Autodesk Inventor part; units mm, degrees
ref_plane "YZ Plane" through (0, 0, 0) normal (1, 0, 0) x (0, 1, 0)
ref_plane "XZ Plane" through (0, 0, 0) normal (0, 1, 0) x (-1, 0, 0)
ref_plane "XY Plane" through (0, 0, 0) normal (0, 0, 1) x (1, 0, 0)
sketch "Esboço1" plane through (0, 0, 0) normal (0, 0, 1) x (1, 0, 0)
  line L0 (0, 0) -> (22, 0)
  line L1 (22, 0) -> (22, 20)
  line L2 (22, 20) -> (0, 20)
  line L3 (0, 20) -> (0, 0)
  dimension "d0" = 22
  dimension "d1" = 20
extrude "Extrusão1" add sketch "Esboço1" along normal blind 50
sketch "Esboço2" plane through (0, 0, 0) normal (0, -1, 0) x (1, 0, 0)
  line L0 (0, 0) -> (0, 50)
  line L1 (22, 50) -> (0, 50)
  point P0 (11, 15.5027)
  dimension "d20" = 11
  dimension "d35" = 34.4973
hole "Furo1" at (11, 0, 15.5027) direction (0, 1, 0) diameter 15 end through all
fillet "Arredondamento1" radius 5 4 edges at (22, 10, 0) (0, 10, 0) (0, 10, 50) (22, 10, 50)
sketch "Esboço4" plane through (5, 20, 0) normal (0, 1, 0) x (1, 0, 0)
  line L0 (12, -50) -> (0, -50)
  line L1 (6, -50) -> (6, -25)
  line L2 (1, -50) -> (11, -50)
  line L3 (11, -50) -> (11, -25)
  line L4 (11, -25) -> (1, -25)
  line L5 (1, -25) -> (1, -50)
  line L6 (1, -50) -> (11, -25) construction
  line L7 (11, -50) -> (1, -25) construction
  point P0 (-5, 0)
  point P1 (6, -37.5)
  dimension "d22" = 25
  dimension "d23" = 10
extrude "Extrusão2" cut sketch "Esboço4" against normal through all
sketch "Esboço5" plane through (16, 20, 25) normal (-1, 0, 0) x (0, 0, 1)
  line L0 (25, -20) -> (25, 0)
  point P0 (-25, -20)
  point P1 (20, -10)
  point P2 (10, -10)
  dimension "d33" = 5
  dimension "d34" = 10
hole "Furo3" at (16, 10, 45) at (16, 10, 35) direction (1, 0, 0) diameter 3 end through all both
properties part number "Base 1 LMU8_3DPrint"
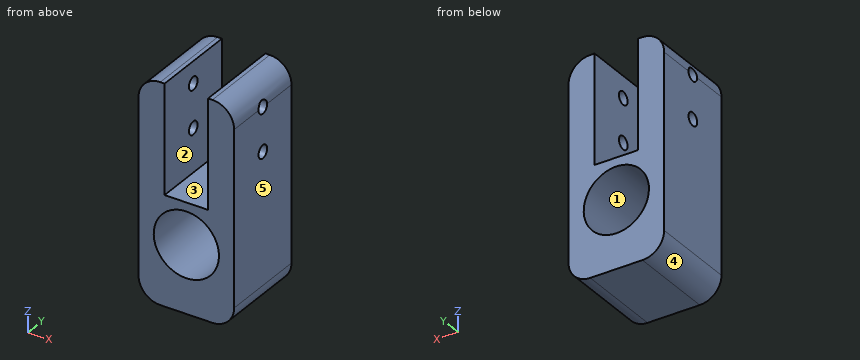
Check sheet for the modelled part. Datum: model origin and axes. Units: mm. Face numbers are marked on the shaded views. A direction names the side the tool comes from. Round coordinates to 2 decimals unless told otherwise and drop trailing zeros. Loops run counter-clockwise (first coordinate to the right, second up) from the corner with the lowest first, then second, coordinate; pieces in that order, holes last. Notation, with made-up numbers: M 23.25,58 L 59.25,58 A11 cw 59.25,63 Z; hole C 20,-36.5 d2. An arc over 180 degrees is marked long. One line per item, written item: value.
(1) Sectioned sample at A-A, the plane x = 11. Record the cut outline in (y, z), then the cut area to 3 significant figures.
Computed values:
outline: M 0,0 L 20,0 L 20,8 L 0,8 Z; M 0,23 L 20,23 L 20,25 L 0,25 Z
area: 200 mm^2
(2) Sectioned sample at B-B, the plane z = 42. Record the cut outline in (x, y), then the cut area to 3 significant figures.
Computed values:
outline: M 0,0 L 6,0 L 6,20 L 0,20 Z; M 16,0 L 22,0 L 22,20 L 16,20 Z
area: 240 mm^2
(3) Sectioned sample at C-C, the plane y = 18.5. Record the cut outline in (x, z).
Computed values:
outline: M 0,5 A5 ccw 5,0 L 17,0 A5 ccw 22,5 L 22,45 A5 ccw 17,50 L 16,50 L 16,25 L 6,25 L 6,50 L 5,50 A5 ccw 0,45 Z; hole C 11,15.5 d15
(4) Access from +Z, -Z, +X, -X, +Y, -Y to the whole of each face (thin tool, end or side, straight path). Record for the marked faces 1 and 2.
Computed values:
face 1: +Y, -Y
face 2: +Z, +Y, -Y
(5) Release check for a two-part mould opening along X. For the marked faces 3, 4 and 5 record: +X half, -X half, draft (parallel to the pull), parting line (faces both ways), or undercut.
Computed values:
face 3: undercut
face 4: -X half
face 5: +X half
(6) Thickness scan on line 1 (X direction, y = 12, z = 28.5); line 2 (Z direction, x = 1.25, y = 10); line 3 (Z direction, x = 20.25, y = 10). Record the ranges inside material, lowest first.
Computed values:
line 1: x = 0 to 6, 16 to 22
line 2: z = 1.69 to 33.5, 36.5 to 43.5, 46.5 to 48.31
line 3: z = 1.2 to 33.5, 36.5 to 43.5, 46.5 to 48.8
(7) Sectioned sample at D-D, the plane z = 35. Record the cut outline in (x, y).
Computed values:
outline: M 0,0 L 6,0 L 6,8.5 L 0,8.5 Z; M 0,11.5 L 6,11.5 L 6,20 L 0,20 Z; M 16,0 L 22,0 L 22,8.5 L 16,8.5 Z; M 16,11.5 L 22,11.5 L 22,20 L 16,20 Z
(8) Depth check by flat-ended pin: pin 1 Ø8 at (x, y) = (11.5, 6.5) entering from +Z. Enter the tip coordinate at first touch or a pass-through.
Computed values:
pin 1: stops at z = 25
